from build123d import *

# Parameters (mm, degrees)
F0_R     = 11
F1_DEPTH = 8


with BuildPart() as f1:
    # F0 (on Top) → F1 (new body)
    with BuildSketch(Plane.XY):
        with BuildLine():
            ThreePointArc((9.526279, 19.5), (0, 14), (-9.526279, 19.5))
            ThreePointArc((-9.526279, 19.5), (-33.774991, 19.5), (-21.650635, -1.5))
            ThreePointArc((-21.650635, -1.5), (-12.124356, -7), (-12.124356, -18))
            ThreePointArc((-12.124356, -18), (0, -39), (12.124356, -18))
            ThreePointArc((12.124356, -18), (12.124356, -7), (21.650635, -1.5))
            ThreePointArc((21.650635, -1.5), (33.774991, 19.5), (9.526279, 19.5))
        make_face()
        Polygon((3.57134, -15.857852), (9.703002, -23.521797), (6.131662, -32.663945), (-3.57134, -34.142148), (-9.703002, -26.478203), (-6.131662, -17.336055), align=None, mode=Mode.SUBTRACT)
        Polygon((-16.743158, 21), (-11.835681, 12.5), (-16.743158, 4), (-26.558112, 4), (-31.46559, 12.5), (-26.558112, 21), align=None, mode=Mode.SUBTRACT)
        Circle(F0_R, mode=Mode.SUBTRACT)
        Polygon((16.435203, 20.814602), (26.243575, 21.173997), (31.459007, 12.859396), (26.866067, 4.185398), (17.057695, 3.826003), (11.842263, 12.140604), align=None, mode=Mode.SUBTRACT)
    extrude(amount=F1_DEPTH)


solid = f1.part
Design review of the part built by this model. Coordinates are the model's own, in mm. A direction names the side the tool comes from. Give positions to 0.01 mm unless a question says otherwise; leave off trailing zeros. Loops run counter-clockwise (first coordinate to the right, second up) from the corner with the lowest first, then second, coordinate; pieces in that order, holes last. Notation, with made-up numbers: (-7, -20) - (1, -20) arc R7 ccw to (1, -14) - close; hole circle Ø1 at (-13, -30). An arc over 180 degrees is marked (long way). Use CSV: the item, a comma, the result in double quotes. Start each with the question number.
1. Add section D-D (x = 20.5). State the section outline as (y, z) points, plus the area to 3 significant figures.
2. Add section A-A (x = 0). State the section outline as (y, z) points.
3. Add section B-B (y = -28). State the section outline as (x, z) points.
4. Add section C-C (y = 16.5). State the section outline as (x, z) points.
5. Insertion check: P1, Ø5, axis at x = -27, y = 11.5, coming from the -Z side; P2, Ø3, axis at x = -0.5, z = 1, coming from the +Y side; P3, Ø2, axis at y = -19.5, z = 2, coming from the +X side. Each pin has a flat end and moves straight along its axis. Give the tip position at first contact, or say it passes through.
6. Machinability: for faces 4 (the flat face through (7.94, -28.03, 3.94)), 5 (the cylindrical face through (12.045, -7.14, 3.944)), which of the approach directions +Z, -Z, +X, -X, +Y, -Y give a long, thin tool a straight path to every point of the face, cutting with its end or side? Answer none if there is none.
7. Wall thickness on L1, parallel to X at y = -3, z = 4.5; L2, parallel to Y at x = -17, z = 6.5; L3, parallel to X at y = -27.5, z = 2.5: over which ranges is each line inside the solid? List them lowest first.
8. Draft analysis for pull direction Y (two halves, no side actions). For faces 1 (the cylindrical face through (0, 14, 4)), 2 (the cylindrical face through (33.975, 19.142, 3.944)), 3 (the flat face through (-14.324, 16.81, 3.944)), state which applies: released by +Y, released by -Y, zero draft, split by the parting line, or undercut.
Results found:
1,outline,"(-1.56, 0) - (3.95, 0) - (3.95, 8) - (-1.56, 8) - close; (20.96, 0) - (26.45, 0) - (26.45, 8) - (20.96, 8) - close"
1,area,"88.0 mm²"
2,outline,"(-39, 0) - (-33.6, 0) - (-33.6, 8) - (-39, 8) - close; (-16.4, 0) - (-11, 0) - (-11, 8) - (-16.4, 8) - close; (11, 0) - (14, 0) - (14, 8) - (11, 8) - close"
3,outline,"(-13.67, 0) - (-8.49, 0) - (-8.49, 8) - (-13.67, 8) - close; (7.95, 0) - (13.67, 0) - (13.67, 8) - (7.95, 8) - close"
4,outline,"(-35.07, 0) - (-29.16, 0) - (-29.16, 8) - (-35.07, 8) - close; (-14.15, 0) - (-6.98, 0) - (-6.98, 8) - (-14.15, 8) - close; (6.98, 0) - (14.15, 0) - (14.15, 8) - (6.98, 8) - close; (29.18, 0) - (35.07, 0) - (35.07, 8) - (29.18, 8) - close"
5,P1,"passes through"
5,P2,"stops at y = 14.18"
5,P3,"stops at x = 13.26"
6,face 4,"+Z, -Z"
6,face 5,"+Z, -Z, +X"
7,L1,"x = -16.11 to -10.58, 10.58 to 16.11"
7,L2,"y = -2.53 to 4, 21 to 25.7"
7,L3,"x = -13.77 to -8.89, 8.15 to 13.77"
8,face 1,"released by +Y"
8,face 2,"split by the parting line"
8,face 3,"undercut"
